Source: CAD feature listing. Evaluate the final solid. Frame: model axes, mm. A direction names the side the tool comes from. Round coordinates to 2 decimals unless told otherwise and drop trailing zeros. Order: outer loops, then holes, each group sorted by start corner. A loop starts at its lowest first (then second) coordinate and runs counter-clockwise, first axis right, second up. Notation, with made-up numbers: (-32, 85) -> (5, 85) arc R20 ccw to (5, 113) -> close; hole circle Ø10 at (62.5, 68.5). An arc over 180 degrees is marked (long way). Write item = value, one per line. Start each with the question number.
(1) Cut plane A-A on x = 46. Return the cut outline in (y, z), then the cut area to 3 significant figures.
(2) Draft query along Y for faces 1 (the face through (14.55, 33.66, 3.13)), 2 (the face through (18.2, 35.7, 4.7)), 3 (the face through (84.2, 160.2, 3.2)). Return one class per face: released by +Y, released by -Y, zero draft, split by the parting line, or undercut.
(3) Cut plane B-B on x = 58.5. Return the cut outline in (y, z).
(4) Ray query, line 1 (X direction, y = 43, z = 4.5); line 2 (X direction, y = 159.5, z = 3); line 3 (Y direction, x = 47, z = 3.5). Return the intervals inside material, ascending.
(5) Contact query for flat-ended pins moving along their axis: pin 1 Ø0.5 at (y, z) = (164.5, 3) entering from +X; pin 2 Ø3 at (x, z) = (41, 2.5) entering from -Y; pin 3 Ø3 at (y, z) = (172.87, 3.18) entering from +X; pin 4 Ø6 at (x, y) = (32.21, 39.51) entering from -Z. Output: stop coordinate, or through.
(6) Reachability of faces 4 (the face through (88.328, 171, 3)), 5 (the face through (55, 93, 6.35)), 6 (the face through (85.154, 171.6, 3.8)), 7 (the face through (90.379, 153.022, 3.131)), 8 (the face through (20.652, 34.216, 3.131)) from +Z, -Z, +X, -X, +Y, -Y: full face, straight path, thin tool, end or side. Return the list, or none.
(7) Cut plane C-C on y = 90.5. Return the cut outline in (x, z), then the cut area to 3 significant figures.
from build123d import *

# Parameters (mm, degrees)
SKETCH1_R                 = 2.159
BOSS_EXTRUDE1_DEPTH       = 6.35
SKETCH2_R                 = 1.8288
CUT_EXTRUDE1_DEPTH        = 127.508450551
SKETCH3_R                 = 0.635
CUT_EXTRUDE2_DEPTH        = 76.033777739
FILLET1_R                 = 1.5875
FILLET2_R                 = 38.1
M3X0_5_TAPPED_HOLE1_D     = 2.5
M3X0_5_TAPPED_HOLE1_DEPTH = 7.50062
M3X0_5_TAPPED_HOLE1_TIP   = 0.751075774


with BuildPart() as part:
    # Sketch1 → Boss-Extrude1 (new body)
    with BuildSketch(Plane.XY):
        with BuildLine():
            Line((15.834722261, 31.434493723), (25.183466494, 36.831993723))
            Line((25.183466494, 36.831993723), (26.929716494, 33.8074))
            Line((26.929716494, 33.8074), (27.78608986, 34.301827393))
            ThreePointArc((27.78608986, 34.301827393), (29.23868298, 34.44834582), (30.311273673, 33.457869357))
            ThreePointArc((30.311273673, 33.457869357), (34.825897026, 33.143744407), (32.428977808, 36.9824))
            ThreePointArc((32.428977808, 36.9824), (30.032058591, 40.821055593), (34.546681944, 40.506930643))
            ThreePointArc((34.546681944, 40.506930643), (34.984344673, 39.889437479), (35.639187691, 39.509928464))
            Line((35.639187691, 39.509928464), (40.774282272, 37.860721969))
            ThreePointArc((40.774282272, 37.860721969), (47.368100791, 42.064756802), (42.017768622, 47.767939879))
            ThreePointArc((42.017768622, 47.767939879), (40.437125748, 48.5456558), (40.301653082, 50.302050149))
            Line((40.301653082, 50.302050149), (87.227692295, 149.642175178))
            ThreePointArc((87.227692295, 149.642175178), (87.739785188, 150.497310852), (88.408996906, 151.235993347))
            Line((88.408996906, 151.235993347), (92.404798917, 154.858512458))
            ThreePointArc((92.404798917, 154.858512458), (93.060884875, 155.23586864), (93.814481006, 155.3061491))
            ThreePointArc((93.814481006, 155.3061491), (96.343832869, 159.058865136), (91.821, 158.9024))
            ThreePointArc((91.821, 158.9024), (87.298167131, 158.745934864), (89.827518994, 162.4986509))
            ThreePointArc((89.827518994, 162.4986509), (91.22159212, 162.932303457), (91.821, 164.263545213))
            Line((91.821, 164.263545213), (91.821, 165.2524))
            Line((91.821, 165.2524), (88.3285, 165.2524))
            Line((88.3285, 165.2524), (88.3285, 176.0474))
            Line((88.3285, 176.0474), (85.1535, 176.0474))
            Line((85.1535, 176.0474), (85.1535, 160.118189826))
            Line((85.1535, 160.118189826), (31.375529243, 46.272861553))
            Line((31.375529243, 46.272861553), (13.294722261, 35.833902774))
            Line((13.294722261, 35.833902774), (15.834722261, 31.434493723))
        make_face()
        with Locations((42.327648174, 42.6974)):
            Circle(SKETCH1_R, mode=Mode.SUBTRACT)
    extrude(amount=BOSS_EXTRUDE1_DEPTH)

    # Sketch2 → Cut-Extrude1 (cut, through all)
    with BuildSketch(Plane(origin=(-9.652854494, 16.719234422, 0), x_dir=(-0.866025404, -0.5, 0), z_dir=(0.5, -0.866025404, 0))):
        with Locations(Location((-32.605518601, -3.175, 0), (0, 0, 180))):  # turned: the seam where the file's is
            Circle(SKETCH2_R)
    extrude(amount=-CUT_EXTRUDE1_DEPTH, mode=Mode.SUBTRACT)

    # Sketch3 → Cut-Extrude2 (cut, through all)
    with BuildSketch(Plane(origin=(88.3285, 0, 0), x_dir=(0, 0, -1), z_dir=(1, 0, 0))):
        with Locations((-3.175, 172.8724)):
            Circle(SKETCH3_R)
    extrude(amount=-CUT_EXTRUDE2_DEPTH, mode=Mode.SUBTRACT)

    # Fillet1
    fillet1_edges = [part.edges().sort_by_distance(p)[0] for p in [
        (88.3285, 165.2524, 3.175),
        (25.183466494, 36.831993723, 3.175),
    ]]
    fillet(fillet1_edges, radius=FILLET1_R)

    # Fillet2
    fillet2_edges = [part.edges().sort_by_distance(p)[0] for p in [
        (31.375529243, 46.272861553, 3.175),
        (85.1535, 160.118189826, 3.175),
    ]]
    fillet(fillet2_edges, radius=FILLET2_R)

    # M3x0.5 Tapped Hole1
    with Locations(Plane.ZY.offset(-85.1535)):
        with Locations((3.175, 172.8724)):
            Hole(M3X0_5_TAPPED_HOLE1_D / 2, depth=M3X0_5_TAPPED_HOLE1_DEPTH)
            with Locations((0, 0, -(M3X0_5_TAPPED_HOLE1_DEPTH + M3X0_5_TAPPED_HOLE1_TIP / 2))):  # 118° drill point
                Cone(0, M3X0_5_TAPPED_HOLE1_D / 2, M3X0_5_TAPPED_HOLE1_TIP, mode=Mode.SUBTRACT)


solid = part.part
Evaluation:
q1.outline = (39.19, 0) -> (46.21, 0) -> (46.21, 6.35) -> (39.19, 6.35) -> close; (62.37, 0) -> (77.23, 0) -> (77.23, 6.35) -> (62.37, 6.35) -> close
q1.area = 139 mm^2
q2.face_1 = released by -Y
q2.face_2 = undercut
q2.face_3 = released by +Y
q3.outline = (88.83, 0) -> (103.69, 0) -> (103.69, 6.35) -> (88.83, 6.35) -> close
q4.line_1 = 25.09 to 40.19, 44.47 to 47.4
q4.line_2 = 84.03 to 87.02, 92.21 to 96.03
q4.line_3 = 40.7 to 44.69, 64.48 to 79.35
q5.pin_1 = 91.82
q5.pin_2 = 37.62
q5.pin_3 = 88.33
q5.pin_4 = 0
q6.face_4 = +Z, -Z, +X, +Y
q6.face_5 = +Z, +X, -X, +Y, -Y
q6.face_6 = +Z, -Z, -X, +Y
q6.face_7 = +Z, -Z, +X, -Y
q6.face_8 = +Z, -Z, -Y
q7.outline = (52.27, 0) -> (59.29, 0) -> (59.29, 6.35) -> (52.27, 6.35) -> close
q7.area = 44.6 mm^2
